Autodesk Inventor part; units mm, degrees
ref_plane "YZ Plane" through (0, 0, 0) normal (1, 0, 0) x (0, 1, 0)
ref_plane "XZ Plane" through (0, 0, 0) normal (0, 1, 0) x (-1, 0, 0)
ref_plane "XY Plane" through (0, 0, 0) normal (0, 0, 1) x (1, 0, 0)
sketch "Sketch1" plane through (0, 0, 0) normal (0, 1, 0) x (-1, 0, 0)
  circle A0 centre (0, 0) radius 15.6
  circle A1 centre (0, 0) radius 10
  dimension "d0" = 31.2
  dimension "d1" = 20
extrude "Extrusion1" add sketch "Sketch1" along normal mid plane 13.2
fillet "Fillet1" radius 1 2 edges at (15.6, 6.6, 0) (15.6, -6.6, 0)
fillet "Fillet2" radius 1 2 edges at (10, 6.6, 0) (10, -6.6, 0)
properties part number "Opona"
Could you check a few things on this model? Use its own coordinates, in mm. Give positions to 0.01 mm unless a question says otherwise; leave off trailing zeros. Order: outer loops, then holes, each group sorted by start corner. A loop starts at its lowest first (then second) coordinate and runs counter-clockwise, first axis right, second up. Notation, with made-up numbers: (87, -29.5) -> (97, -29.5) arc R15 ccw to (97, -14.5) -> close; hole circle Ø8 at (-25, 3). An arc over 180 degrees is marked (long way). Answer in a Markdown table with one row per item. Add a question column.
Item 1: Imagine slicing it at B-B (z = 0). List the corners of the cut face in (x, y) for me.
Item 2: We'd pull the mould along Z, two halves only. Please class faces 1 (the cylindrical face through (2.17, -0.08, 9.76)), 2 (the flat face through (-2, 6.6, 11)), 3 (the cylindrical face through (11.5, 0.08, 10.54)): pulls with the +Z half, pulls with the -Z half, needs draft (parallel to the pull), parting line crosses it, or undercut.
Item 3: Imagine slicing it at C-C (y = 3.5). List the corners of the cut face in (x, z) for me.
Item 4: Please list where these lines run through material, in increasing order: probe 1 along Z at (x, y) = (0, 1.75); probe 2 along Z at (x, y) = (-5, -1); probe 3 along X at (y, z) = (1.5, -8.5).
Item 5: Imagine slicing it at A-A (x = 0). List the corners of the cut face in (y, z) for me.
Item 6: I'm going to push flat-ended pins straight in: P1, Ø3, axis at x = 2, y = -1, coming from the -Z side; P2, Ø16, axis at x = 0, z = 0, coming from the +Y side; P3, Ø6, axis at y = 2.5, z = -4, coming from the +X side; P4, Ø5, axis at y = 5, z = 12, coming from the -X side. Where does each tip first touch, or does it pass through?
Result:
| question | item | result |
|---|---|---|
| 1 | outline | (-15.6, -5.6) arc R1 ccw to (-14.6, -6.6) -> (-11, -6.6) arc R1 ccw to (-10, -5.6) -> (-10, 5.6) arc R1 ccw to (-11, 6.6) -> (-14.6, 6.6) arc R1 ccw to (-15.6, 5.6) -> close; (10, -5.6) arc R1 ccw to (11, -6.6) -> (14.6, -6.6) arc R1 ccw to (15.6, -5.6) -> (15.6, 5.6) arc R1 ccw to (14.6, 6.6) -> (11, 6.6) arc R1 ccw to (10, 5.6) -> close |
| 2 | face 1 | undercut |
| 2 | face 2 | needs draft |
| 2 | face 3 | parting line crosses it |
| 3 | outline | circle Ø31.2 at (0, 0); hole circle Ø20 at (0, 0) |
| 4 | probe 1 | -15.6 to -10, 10 to 15.6 |
| 4 | probe 2 | -14.78 to -8.66, 8.66 to 14.78 |
| 4 | probe 3 | -13.08 to -5.27, 5.27 to 13.08 |
| 5 | outline | (-6.6, -14.6) arc R1 ccw to (-5.6, -15.6) -> (5.6, -15.6) arc R1 ccw to (6.6, -14.6) -> (6.6, -11) arc R1 ccw to (5.6, -10) -> (-5.6, -10) arc R1 ccw to (-6.6, -11) -> close; (-6.6, 11) arc R1 ccw to (-5.6, 10) -> (5.6, 10) arc R1 ccw to (6.6, 11) -> (6.6, 14.6) arc R1 ccw to (5.6, 15.6) -> (-5.6, 15.6) arc R1 ccw to (-6.6, 14.6) -> close |
| 6 | P1 | z = -15.59 |
| 6 | P2 | through |
| 6 | P3 | x = 15.57 |
| 6 | P4 | x = -12.37 |
